For this review, take the finished solid that the model builds, in its own axes (mm). Face numbers are marked on the shaded views. A direction names the side the tool comes from. Give positions to 0.01 mm unless a question says otherwise; leave off trailing zeros. Order: outer loops, then holes, each group sorted by start corner. A loop starts at its lowest first (then second) coordinate and runs counter-clockwise, first axis right, second up. Notation, with made-up numbers: (49, 75) - (64, 75) arc R26 cw to (64, 92) - close; hole circle Ø2 at (8.5, 75). An arc over 180 degrees is marked (long way). Use a Markdown table: item, result. Add a question column.
1) We need section C-C on z = -1.55. Write out the cut boundary in (x, y).
2) We need section A-A on x = 0. Write out the cut boundary in (y, z).
3) Wall thickness on L1, parallel to Y at x = 0, z = 0.15; L2, parallel to Y at x = 0, z = 1.05; L3, parallel to Z at x = -8, y = -2: over which ranges is each line inside the solid? List them lowest first.
4) We need section B-B on y = 0.75. Write out the cut boundary in (x, z), then the cut area to 3 significant figures.
5) Mouldability with a two-part tool opening along X and no side actions: class the marked faces 4, 5 and 6 as released by +X, released by -X, zero draft, split by the parting line, or undercut.
6) Machinability: for the marked faces 1, 2 and 3, which of the approach directions +Z, -Z, +X, -X, +Y, -Y give a long, thin tool a straight path to every point of the face, cutting with its end or side? Answer none if there is none.
7) Clearance check with flat-ended pins moving along their axes: P1, Ø3, axis at x = 0, y = 0, coming from the +Z side; P2, Ø3, axis at x = 0, y = 0, coming from the -Z side; P3, Ø1.5, axis at x = -5, z = -0.5, coming from the -Y side. State where each tip first meets the part, or that it passes through.
8) We need section D-D on x = -14.5. Write out the cut boundary in (y, z).
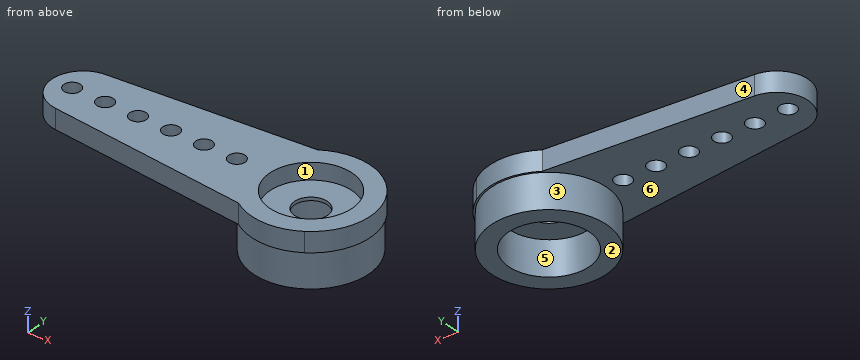
```python
from build123d import *
from build123d.topology import SkipClean

# Parameters (mm, degrees)
BOSS_EXTRUDE1_DEPTH = 1.2
SKETCH2_R           = 3.5
BOSS_EXTRUDE2_DEPTH = 2.1
SKETCH3_R           = 2.5
CUT_EXTRUDE1_DEPTH  = 1
SKETCH4_R           = 1
CUT_EXTRUDE2_DEPTH  = 19.149516235
SKETCH6_R           = 2.45
CUT_EXTRUDE3_DEPTH  = 2.1
SKETCH8_R           = 0.5
CUT_EXTRUDE5_DEPTH  = 19.303140156
CUT_EXTRUDE6_DEPTH  = 10
CUT_EXTRUDE7_DEPTH  = 10


with BuildPart() as part:
    # Sketch1 → Boss-Extrude1 (new body)
    with BuildSketch(Plane.XY):
        with BuildLine():
            Line((-2, -6.75), (-2, -3))
            Line((-2, -3), (-14, -1.9))
            ThreePointArc((-14, -1.9), (-15.733799273, 0), (-14, 1.9))
            Line((-14, 1.9), (-2, 3))
            Line((-2, 3), (-2, 6.75))
            ThreePointArc((-2, 6.75), (0, 8.75), (2, 6.75))
            Line((2, 6.75), (2, 3))
            Line((2, 3), (14, 1.9))
            ThreePointArc((14, 1.9), (15.733799273, 0), (14, -1.9))
            Line((14, -1.9), (2, -3))
            Line((2, -3), (2, -6.75))
            ThreePointArc((2, -6.75), (0, -8.75), (-2, -6.75))
        make_face()
    extrude(amount=BOSS_EXTRUDE1_DEPTH)

    # Sketch2 → Boss-Extrude2 (add)
    with BuildSketch(Plane(origin=(0, 0, 0), x_dir=(-1, 0, 0), z_dir=(0, 0, -1))):
        Circle(SKETCH2_R)
    extrude(amount=BOSS_EXTRUDE2_DEPTH)

    # Sketch3 → Cut-Extrude1 (cut)
    with BuildSketch(Plane.XY.offset(1.2)):
        Circle(SKETCH3_R)
    extrude(amount=-CUT_EXTRUDE1_DEPTH, mode=Mode.SUBTRACT)

    # Sketch4 → Cut-Extrude2 (cut, through all)
    with BuildSketch(Plane.XY.offset(0.2)):
        Circle(SKETCH4_R)
    extrude(amount=-CUT_EXTRUDE2_DEPTH, mode=Mode.SUBTRACT)

    # Sketch6 → Cut-Extrude3 (cut)
    with BuildSketch(Plane(origin=(0, 0, -2.1), x_dir=(-1, 0, 0), z_dir=(0, 0, -1))):
        Circle(SKETCH6_R)
    extrude(amount=-CUT_EXTRUDE3_DEPTH, mode=Mode.SUBTRACT)

    # Sketch8 → Cut-Extrude5 (cut, through all)
    with BuildSketch(Plane.XY.offset(1.2)):
        with Locations((-4.5, 0)):
            Circle(SKETCH8_R)
        with Locations((-6.5, 0)):
            Circle(SKETCH8_R)
        with Locations((-8.5, 0)):
            Circle(SKETCH8_R)
        with Locations((-10.5, 0)):
            Circle(SKETCH8_R)
        with Locations((-12.5, 0)):
            Circle(SKETCH8_R)
        with Locations((-14.5, 0)):
            Circle(SKETCH8_R)
    extrude(amount=-CUT_EXTRUDE5_DEPTH, mode=Mode.SUBTRACT)

    # Sketch10 → Cut-Extrude6 (cut)
    with BuildSketch(Plane(origin=(0, 0, 0), x_dir=(-1, 0, 0), z_dir=(0, 0, -1))):
        with BuildLine():
            Line((-2, 3), (-3.5, 8.058048999))
            Line((-3.5, 8.058048999), (0.410688034, 10.263711762))
            Line((0.410688034, 10.263711762), (4.972399658, 6.328608878))
            Line((4.972399658, 6.328608878), (2, 3))
            ThreePointArc((2, 3), (0, 3.605551275), (-2, 3))
        make_face()
        with BuildLine():
            Line((-2, -3), (-3.79905406, -6.652770289))
            Line((-3.79905406, -6.652770289), (-0.630835306, -10.284036399))
            Line((-0.630835306, -10.284036399), (2.565835598, -9.787591171))
            Line((2.565835598, -9.787591171), (3.731558209, -4.826385145))
            Line((3.731558209, -4.826385145), (2, -3))
            ThreePointArc((2, -3), (0, -3.605551275), (-2, -3))
        make_face()
    extrude(amount=-CUT_EXTRUDE6_DEPTH, mode=Mode.SUBTRACT)

    # Sketch12 → Cut-Extrude7 (cut)
    with SkipClean():  # the faces are left unmerged after this step: merging them gives an invalid solid
        with BuildSketch(Plane(origin=(0, 0, 0), x_dir=(-1, 0, 0), z_dir=(0, 0, -1))):
            with BuildLine():
                Line((-14, 1.9), (-2, 3))
                ThreePointArc((-2, 3), (-3.605551275, 0), (-2, -3))
                Line((-2, -3), (-14, -1.9))
                ThreePointArc((-14, -1.9), (-15.733799273, 0), (-14, 1.9))
            make_face()
        extrude(amount=-CUT_EXTRUDE7_DEPTH, mode=Mode.SUBTRACT)


solid = part.part
```
Checked values:
| question | item | result |
|---|---|---|
| 1 | outline | circle Ø7 at (0, 0); hole circle Ø4.9 at (0, 0) |
| 2 | outline | (-3.61, 0) - (-3.5, 0) - (-3.5, -2.1) - (-2.45, -2.1) - (-2.45, 0) - (-1, 0) - (-1, 0.2) - (-2.5, 0.2) - (-2.5, 1.2) - (-3.61, 1.2) - close; (1, 0) - (2.45, 0) - (2.45, -2.1) - (3.5, -2.1) - (3.5, 0) - (3.61, 0) - (3.61, 1.2) - (2.5, 1.2) - (2.5, 0.2) - (1, 0.2) - close |
| 3 | L1 | -3.61 to -1, 1 to 3.61 |
| 3 | L2 | -3.61 to -2.5, 2.5 to 3.61 |
| 3 | L3 | 0 to 1.2 |
| 4 | outline | (-15.58, 0) - (-3.42, 0) - (-3.42, -2.1) - (-2.33, -2.1) - (-2.33, 0) - (-0.66, 0) - (-0.66, 0.2) - (-2.38, 0.2) - (-2.38, 1.2) - (-15.58, 1.2) - close; (0.66, 0) - (2.33, 0) - (2.33, -2.1) - (3.42, -2.1) - (3.42, 0) - (3.53, 0) - (3.53, 1.2) - (2.38, 1.2) - (2.38, 0.2) - (0.66, 0.2) - close |
| 4 | area | 22.5 mm² |
| 5 | face 4 | released by -X |
| 5 | face 5 | undercut |
| 5 | face 6 | zero draft |
| 6 | face 1 | +Z |
| 6 | face 2 | -Z, +X, -X, +Y, -Y |
| 6 | face 3 | -Z |
| 7 | P1 | z = 0.2 |
| 7 | P2 | z = 0 |
| 7 | P3 | y = -2.78 |
| 8 | outline | (-1.78, 0) - (-0.5, 0) - (-0.5, 1.2) - (-1.78, 1.2) - close; (0.5, 0) - (1.78, 0) - (1.78, 1.2) - (0.5, 1.2) - close |
